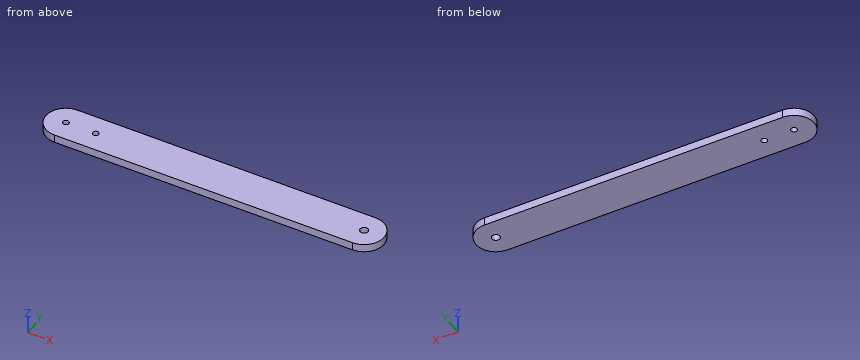
```python
from build123d import *

# Parameters (mm, degrees)
ESQUISSE1_W        = 170
ESQUISSE1_H        = 20
ESQUISSE1_R        = 1.5
ESQUISSE1_R_2      = 2
BOSS_EXTRU_1_DEPTH = 4
CONG_1_RADIUS      = 10
CONG_1_LENGTH      = 4
CONG_2_RADIUS      = 10
CONG_2_LENGTH      = 4


with BuildPart() as part:
    # Esquisse1 → Boss.-Extru.1 (new body)
    with BuildSketch(Plane.XY):
        with Locations((-85, 10)):
            Rectangle(ESQUISSE1_W, ESQUISSE1_H)
        with Locations((-160, 10)):
            Circle(ESQUISSE1_R, mode=Mode.SUBTRACT)
        with Locations((-10, 10)):
            Circle(ESQUISSE1_R_2, mode=Mode.SUBTRACT)
        with Locations((-145, 10)):
            Circle(ESQUISSE1_R, mode=Mode.SUBTRACT)
    extrude(amount=BOSS_EXTRU_1_DEPTH)

    # Congé1: full round fillet: the end face becomes a half cylinder, R = half its width
    cong_1_face = Plane((-170, 10, 2), x_dir=(0, 0, 1), z_dir=(-1, 0, 0))  # on the end face: x along it, z out of the body
    cong_1_slab = cong_1_face.offset(-CONG_1_RADIUS / 2) * Box(CONG_1_LENGTH, 2 * CONG_1_RADIUS, CONG_1_RADIUS, mode=Mode.PRIVATE)  # the body's end, R deep
    cong_1_round = Plane((-160, 10, 2), x_dir=(-1, 0, 0), z_dir=(0, 0, 1)) * Cylinder(CONG_1_RADIUS, CONG_1_LENGTH, mode=Mode.PRIVATE)  # its axis R under the face
    add(cong_1_slab - cong_1_round, mode=Mode.SUBTRACT)

    # Congé2: full round fillet: the end face becomes a half cylinder, R = half its width
    cong_2_face = Plane((0, 10, 2), x_dir=(0, 0, -1), z_dir=(1, 0, 0))  # on the end face: x along it, z out of the body
    cong_2_slab = cong_2_face.offset(-CONG_2_RADIUS / 2) * Box(CONG_2_LENGTH, 2 * CONG_2_RADIUS, CONG_2_RADIUS, mode=Mode.PRIVATE)  # the body's end, R deep
    cong_2_round = Plane((-10, 10, 2), x_dir=(1, 0, 0), z_dir=(0, 0, -1)) * Cylinder(CONG_2_RADIUS, CONG_2_LENGTH, mode=Mode.PRIVATE)  # its axis R under the face
    add(cong_2_slab - cong_2_round, mode=Mode.SUBTRACT)


solid = part.part
```
The listing builds one solid part. Answer for the finished solid, in the listing's coordinates (mm). Coordinates: 2 decimals unless noted, no trailing zeros. Loops run counter-clockwise (first coordinate to the right, second up) from the corner with the lowest first, then second, coordinate; pieces in that order, holes last. Notation, with made-up numbers: (-10.5, -37.75) - (0.5, -37.75) arc R24 ccw to (0.5, -13.75) - close; hole circle Ø1 at (6.5, -9.75). An arc over 180 degrees is marked (long way). Use a Markdown table: item, result. Add a question column.
1) The part is cut by section B-B, the plane z = 2.3. Give the vertices of the cut face in (x, y).
2) Given pin 1 (2.5 mm diameter, centred on x = -145, y = 10, fed in from +Z); pin 2 (1 mm diameter, centred on y = 5.5, z = 2.5, fed in from -X), each flat-ended and moving along its own axis, determine where each tip first touches the part or whether it passes through.
3) Find the intervals of material crossed by line 1 (Y direction, x = -160, z = 2.6); line 2 (X direction, y = 16.5, z = 1.7); line 3 (X direction, y = 12.5, z = 1.2), in increasing order.
4) The part is cut by section C-C, the plane x = -145. Give the vertices of the cut face in (y, z), and give its area (3 significant figures).
5) The part is cut by section A-A, the plane y = 10. Give the vertices of the cut face in (x, z), and give its area (3 significant figures).
Here are the results:
| question | item | result |
|---|---|---|
| 1 | outline | (-160, 0) - (-10, 0) arc R10 ccw to (-10, 20) - (-160, 20) arc R10 ccw to start; hole circle Ø3 at (-160, 10); hole circle Ø3 at (-145, 10); hole circle Ø4 at (-10, 10) |
| 2 | pin 1 | passes through |
| 2 | pin 2 | stops at x = -169.17 |
| 3 | line 1 | y = 0 to 8.5, 11.5 to 20 |
| 3 | line 2 | x = -167.6 to -2.4 |
| 3 | line 3 | x = -169.68 to -0.32 |
| 4 | outline | (0, 0) - (8.5, 0) - (8.5, 4) - (0, 4) - close; (11.5, 0) - (20, 0) - (20, 4) - (11.5, 4) - close |
| 4 | area | 68.0 mm^2 |
| 5 | outline | (-170, 0) - (-161.5, 0) - (-161.5, 4) - (-170, 4) - close; (-158.5, 0) - (-146.5, 0) - (-146.5, 4) - (-158.5, 4) - close; (-143.5, 0) - (-12, 0) - (-12, 4) - (-143.5, 4) - close; (-8, 0) - (0, 0) - (0, 4) - (-8, 4) - close |
| 5 | area | 640 mm^2 |
